from build123d import *

# Parameters (mm, degrees)
F0_R      = 2.54
F1_DEPTH  = 76.2
F3_DEPTH  = 5.08
F4_W      = 5.08
F4_H      = 5.08
F4_W_2    = 2.54
F5_DEPTH  = 1.27
F3_FACE_W = 2.54
F3_FACE_H = 5.08
F6_DEPTH  = 3.81
F7_W      = 1.27
F7_H      = 5.08
F8_DEPTH  = 7.62


with BuildPart() as f1:
    # F0 (on Right) → F1 (new body)
    with BuildSketch(Plane.YZ):
        with Locations((-37.062876, 39.933953)):
            Circle(F0_R)
    extrude(amount=F1_DEPTH)

    # F2 (on face) → F3 (join)
    with BuildSketch(Plane.YZ.offset(76.2)):
        with BuildLine():
            Line((-27.742092, 42.473953), (-37.062876, 42.473953))
            ThreePointArc((-37.062876, 42.473953), (-35.266825, 41.730005), (-34.522876, 39.933953))
            ThreePointArc((-34.522876, 39.933953), (-35.266825, 38.137902), (-37.062876, 37.393953))
            Line((-37.062876, 37.393953), (-27.742092, 37.393953))
            Line((-27.742092, 37.393953), (-27.742092, 42.473953))
        make_face()
        with BuildLine():
            Line((-37.062876, 42.473953), (-37.062876, 39.933953))
            Line((-37.062876, 39.933953), (-37.062876, 37.393953))
            ThreePointArc((-37.062876, 37.393953), (-35.266825, 38.137902), (-34.522876, 39.933953))
            ThreePointArc((-34.522876, 39.933953), (-35.266825, 41.730005), (-37.062876, 42.473953))
        make_face()
        with BuildLine():
            Line((-37.062876, 37.393953), (-37.062876, 39.933953))
            Line((-37.062876, 39.933953), (-37.062876, 42.473953))
            ThreePointArc((-37.062876, 42.473953), (-39.602876, 39.933953), (-37.062876, 37.393953))
        make_face()
    extrude(amount=F3_DEPTH)

    # F4 (on face) → F5 (join)
    with BuildSketch(Plane(origin=(0, -27.742092, 0), x_dir=(-1, 0, 0), z_dir=(0, 1, 0))):
        with Locations((-73.66, 39.933953)):
            Rectangle(F4_W, F4_H)
        with Locations((-77.47, 39.933953)):
            Rectangle(F4_W_2, F4_H)
    extrude(amount=F5_DEPTH)

    # F3_face (on face) → F6 (join)
    with BuildSketch(Plane(origin=(78.74, -27.742092, 39.933953), x_dir=(-1, 0, 0), z_dir=(0, 1, 0))):
        with Locations((-1.27, 0)):
            Rectangle(F3_FACE_W, F3_FACE_H)
    extrude(amount=F6_DEPTH)

    # F7 (on face) → F8 (join)
    with BuildSketch(Plane(origin=(78.74, 0, 0), x_dir=(0, -1, 0), z_dir=(-1, 0, 0))):
        with Locations((24.567092, 39.933953)):
            Rectangle(F7_W, F7_H)
    extrude(amount=F8_DEPTH)


solid = f1.part
The model under review builds one solid part; all positions refer to its coordinate system, in mm. A direction names the side the tool comes from. Give positions to 0.01 mm unless a question says otherwise; leave off trailing zeros. Loops run counter-clockwise (first coordinate to the right, second up) from the corner with the lowest first, then second, coordinate; pieces in that order, holes last. Notation, with made-up numbers: (-17.75, -6.5) -> (31.25, -6.5) arc R24 cw to (31.25, 21.5) -> close; hole circle Ø9 at (58.25, -33.5). An arc over 180 degrees is marked (long way). Answer as a JSON object with one key per item and string values. Group by question number.
Q1. Take a section at B-B (z = 38.8). Write out the cut boundary in (x, y), plus the area to 3 significant figures.
Q2. Insertion check: pin 1 (1.5 mm diameter, centred on y = -25.5, z = 38.5, fed in from -X); pin 2 (2.5 mm diameter, centred on x = 73, z = 39.5, fed in from -Y); pin 3 (3 mm diameter, centred on x = 44, z = 40, fed in from +Y). Each pin has a flat end and moves straight along its axis. Give the tip position at first contact, or say it passes through.
Q3. Draft analysis for pull direction Y (two halves, no side actions). For faces 5 (the flat face through (78.74, -26, 40)), 6 (the flat face through (75, -26.472, 40)), 7 (the flat face through (76, -23.932, 40)), 8 (the flat face through (77, -30, 42.474)), state which applies: pulls with the +Y half, pulls with the -Y half, needs draft (parallel to the pull), parting line crosses it, or undercut.
Q4. Take a section at D-D (x = 15). Write out the cut boundary in (y, z), plus the area to 3 significant figures.
Q5. Tool access review of faces 1 (the flat face through (71.12, -25, 40)), 2 (the flat face through (0, -37, 40)), 3 (the flat face through (74, -27.742, 40)), 4 (the cylindrical face through (40.07, -39.08, 38.39)): name each direction out of +Z, -Z, +X, -X, +Y, -Y from which nothing blocks a thin tool from reaching the whole face with its end or side.
Q6. Take a section at A-A (x = 73). Write out the cut boundary in (y, z), plus the area to 3 significant figures.
Q7. Take a section at C-C (y = -35.5). Write out the cut boundary in (x, z).
Q8. Wall thickness on line 1 along X through (y, z) = (-30.75, 37.8); line 2 along X through (y, z) = (-26, 40.55); line 3 along Y through (x, z) = (43.5, 42.1): over which ranges is each line inside the solid? List them lowest first.
Answer below:
{
 "1": {"outline": "(0, -39.34) -> (81.28, -39.34) -> (81.28, -23.93) -> (71.12, -23.93) -> (71.12, -25.2) -> (78.74, -25.2) -> (78.74, -26.47) -> (71.12, -26.47) -> (71.12, -27.74) -> (76.2, -27.74) -> (76.2, -34.79) -> (0, -34.79) -> close", "area": "434 mm2"},
 "2": {"pin 1": "stops at x = 71.12", "pin 2": "stops at y = -39.6", "pin 3": "stops at y = -34.52"},
 "3": {"face 5": "undercut", "face 6": "undercut", "face 7": "pulls with the +Y half", "face 8": "needs draft"},
 "4": {"outline": "circle Ø5.08 at (-37.06, 39.93)", "area": "20.3 mm2"},
 "5": {"face 1": "+Z, -Z, -X, +Y", "face 2": "+Z, -Z, -X, +Y, -Y", "face 3": "+Z, -Z, -X", "face 4": "-X"},
 "6": {"outline": "circle Ø5.08 at (-37.06, 39.93); (-27.74, 37.39) -> (-26.47, 37.39) -> (-26.47, 42.47) -> (-27.74, 42.47) -> close; (-25.2, 37.39) -> (-23.93, 37.39) -> (-23.93, 42.47) -> (-25.2, 42.47) -> close", "area": "33.2 mm2"},
 "7": {"outline": "(0, 37.93) -> (76.2, 37.93) -> (76.2, 37.39) -> (81.28, 37.39) -> (81.28, 42.47) -> (76.2, 42.47) -> (76.2, 41.94) -> (0, 41.94) -> close"},
 "8": {"line 1": "x = 76.2 to 81.28", "line 2": "x = 78.74 to 81.28", "line 3": "y = -38.39 to -35.74"}
}
